Here's the drawing with two shaded views (mm, measured from the low corner). I have some questions. Coordinates: 2 decimals unless noted, no trailing zeros. Write each loop counter-clockwise with the first axis right and the second up, starting at its lowest first coordinate (ties: lowest second). Pieces come first, ordered by that corner, then holes. Notation, with made-up numbers: (9.25, -17.5) - (66.25, -17.5) arc R14 cw to (66.25, -7.5) - close; hole circle Ø10 at (82, 35). An arc over 180 degrees is marked (long way). Answer in a Markdown table with one row per item. Add a question column.
Item 1: If I drill on probe 1 along Z at (x, y) = (14.5, 1.3); probe 2 along X at (y, z) = (0.25, 35.5); probe 3 along X at (y, z) = (0.4, 29), over which ranges is the centre line in solid material (lowest first)? Write a range as from..to.
Item 2: Imagine slicing it at A-A (x = 23.25). Please give me the cut outline in (y, z).
Item 3: I'm going to push a flat-ended pin straight in: pin 1 (1 mm diameter, centred on x = 10, y = 2, fed in from -Z). Where does the tip first touch, or does it pass through?
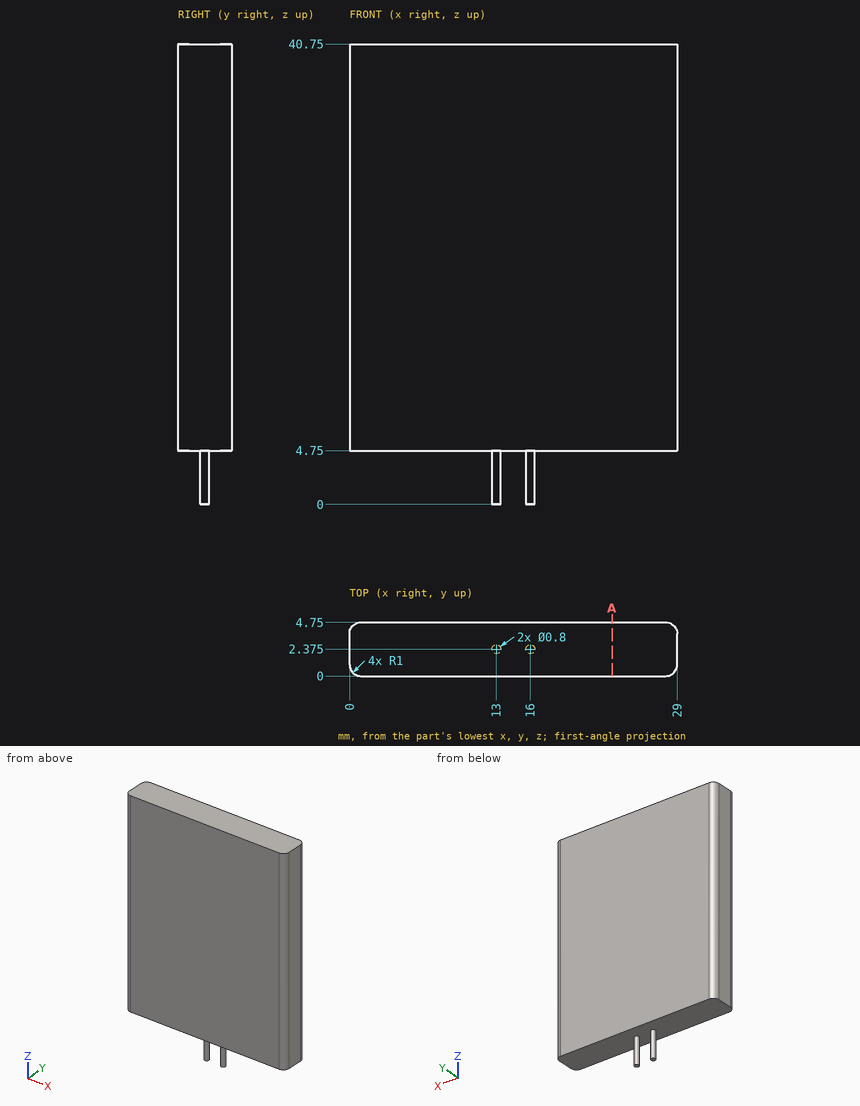
Here are the results:
| question | item | result |
|---|---|---|
| 1 | probe 1 | z = 4.75..40.75 |
| 1 | probe 2 | x = 0.34..28.66 |
| 1 | probe 3 | x = 0.2..28.8 |
| 2 | outline | (0, 4.75) - (4.75, 4.75) - (4.75, 40.75) - (0, 40.75) - close |
| 3 | pin 1 | stops at z = 4.75 |
